from build123d import *

# Parameters (mm, degrees)
F0_R         = 1.8
F0_R_2       = 13.5
F0_W         = 20.1372796029
F0_H         = 13.5
F1_DEPTH     = 2
F2_W         = 3
F2_H         = 33.5
F3_DEPTH     = 27
F4_W         = 16.1372796029
F4_H         = 3
F5_DEPTH     = 25
F6_R         = 1.8
F6_W         = 4
F6_H         = 11
F7_DEPTH     = 25
F8_SIZE      = 25
F9_SIZE      = 14
F10_R        = 5
F11_T1_DEPTH = 2
F11_T3_DEPTH = 32


# Not quite as in the source:
# - a fillet or chamfer that OpenCascade refuses, or shapes differently, is made with other operations: its cross-section is extruded or revolved along the edge and cut away or added


with BuildPart() as f1:
    # F0 (on Top) → F1 (new body)
    with BuildSketch(Plane.XY):
        Polygon((21.15, -21.15), (21.15, 21.15), (-21.15, 21.15), (-21.15, -1.15), (-21.15, -21.15), align=None)
        with Locations((-15.5, -15.5)):
            Circle(F0_R, mode=Mode.SUBTRACT)
        with Locations((15.5, -15.5)):
            Circle(F0_R, mode=Mode.SUBTRACT)
        with Locations((-15.5, 15.5)):
            Circle(F0_R, mode=Mode.SUBTRACT)
        Circle(F0_R_2, mode=Mode.SUBTRACT)
        with Locations((15.5, 15.5)):
            Circle(F0_R, mode=Mode.SUBTRACT)
        Polygon((-21.15, -21.15), (-21.15, -1.15), (-41.3, -1.15), (-41.3, -21.15), (-21.1627203971, -21.15), align=None)
        with Locations((-31.2313601986, -27.9)):
            Rectangle(F0_W, F0_H)
    extrude(amount=F1_DEPTH)

    # F2 (on Top) → F3 (join)
    with BuildSketch(Plane.XY):
        with Locations((-23.6627203971, -17.9)):
            Rectangle(F2_W, F2_H)
    extrude(amount=F3_DEPTH)

    # F4 (on face) → F5 (join)
    with BuildSketch(Plane.XY.offset(2)):
        with Locations((-33.2313601986, -33.15)):
            Rectangle(F4_W, F4_H)
    extrude(amount=F5_DEPTH)

    # F6 (on face) → F7 (cut)
    with BuildSketch(Plane(origin=(0, -31.65, 0), x_dir=(-1, 0, 0), z_dir=(0, 1, 0))):
        with Locations((35.5, 14.5)):
            Circle(F6_R)
        with Locations((35.5, 5.5)):
            Circle(F6_R)
        with Locations((35.5, 23.5)):
            Circle(F6_R)
        with Locations((28.2, 14.5)):
            Rectangle(F6_W, F6_H)
    extrude(amount=-F7_DEPTH, mode=Mode.SUBTRACT)

    # F8
    f8_edges = [f1.edges().sort_by_distance(p)[0] for p in [
        (-23.66272, -1.15, 27),
    ]]
    chamfer(f8_edges, length=F8_SIZE)

    # F9
    f9_edges = [f1.edges().sort_by_distance(p)[0] for p in [
        (-41.3, -1.15, 1),
    ]]
    chamfer(f9_edges, length=F9_SIZE)

    # F10
    f10_edges = [f1.edges().sort_by_distance(p)[0] for p in [
        (-41.3, -15.15, 1),
        (-27.3, -1.15, 1),
        (-21.16272, -34.65, 1),
        (-41.3, -33.15, 27),
    ]]
    fillet(f10_edges, radius=F10_R)

    # F11: fillet of radius 6 on 5 edges, made by hand

    # F11_s2 → F11_t1 (join)
    with BuildSketch(Plane.XY):
        with BuildLine():
            ThreePointArc((-26.1021448299, -1.2268404777), (-22.5517867046, 0.826546392), (-21.15, 4.6809509491))
            Line((-21.15, 4.6809509491), (-20.55, 4.6809509491))
            Line((-20.55, 4.6809509491), (-20.55, -1.15))
            Line((-20.55, -1.15), (-21.15, -1.75))
            ThreePointArc((-21.15, -1.75), (-25.2289321881, -1.75), (-25.9973593129, -1.8176196204))
            Line((-25.9973593129, -1.8176196204), (-26.1021448299, -1.2268404777))
        make_face()
        with BuildLine():
            ThreePointArc((-15.1627203971, -21.15), (-19.4053610842, -22.9073593129), (-21.1627203971, -27.15))
            Line((-21.1627203971, -27.15), (-21.1627203971, -21.15))
            Line((-21.1627203971, -21.15), (-15.1627203971, -21.15))
        make_face()
    extrude(amount=F11_T1_DEPTH)

    # F11_s4 → F11_t3 (cut)
    with BuildSketch(Plane.XY.offset(-15)):
        with BuildLine():
            ThreePointArc((21.15, -15.15), (19.3926406871, -19.3926406871), (15.15, -21.15))
            Line((15.15, -21.15), (21.15, -21.15))
            Line((21.15, -21.15), (21.15, -15.15))
        make_face()
        with BuildLine():
            ThreePointArc((15.15, 21.15), (19.3926406871, 19.3926406871), (21.15, 15.15))
            Line((21.15, 15.15), (21.15, 21.15))
            Line((21.15, 21.15), (15.15, 21.15))
        make_face()
        with BuildLine():
            ThreePointArc((-21.15, 15.15), (-19.3926406871, 19.3926406871), (-15.15, 21.15))
            Line((-15.15, 21.15), (-21.15, 21.15))
            Line((-21.15, 21.15), (-21.15, 15.15))
        make_face()
    extrude(amount=F11_T3_DEPTH, mode=Mode.SUBTRACT)


solid = f1.part
Here's how the part is built. I have some questions about the finished solid (model axes, mm). A direction names the side the tool comes from. Coordinates: 2 decimals unless noted, no trailing zeros. Write each loop counter-clockwise with the first axis right and the second up, starting at its lowest first coordinate (ties: lowest second). Pieces come first, ordered by that corner, then holes.
Item 1: I want a section at C-C on x = -35.5. Write out the boundary of the cut face in (y, z).
Item 2: Will these pins go through, and if not, where does the flat tip stop? pin 1 (5 mm diameter, centred on x = -5.5, y = -24.5, fed in from +Z); pin 2 (0.6 mm diameter, centred on y = 8, z = 1, fed in from -X); pin 3 (2.5 mm diameter, centred on y = -33, z = 13, fed in from +X); pin 4 (6 mm diameter, centred on x = -35.5, z = 5.5, fed in from +Y).
Item 3: If we mould it in two halves opening along Y, with no side actions, what happens to faces 1 (the cylindrical face through (16.468, -13.982, 0.986)), 2 (the flat face through (-33, -31.65, 14)), 3 (the cylindrical face through (-39.87, -33.13, 25.5))? For each: +Y half, -Y half, draft (parallel to the pull), parting line (faces both ways), or undercut.
Item 4: I want a section at D-D on y = 6. Write out the boundary of the cut face in (x, z), and give its area (3 significant figures).
Item 5: I want a section at A-A on x = 0. Write out the boundary of the cut face in (y, z), and give its area (3 significant figures).
Item 6: On a 3-axis mill with a long thin cutter (end or side, diameter ignored), from which of +Z, -Z, +X, -X, +Y, -Y can I reach the whole of each face in a straight line? I mean faces 4 (the flat face through (-10, -11, 2)), 5 (the flat face through (-28, -33, 20)), 6 (the flat face through (-21.163, -28, 1)). Say none if no direction works.
Item 7: If I drill on line 1 (Z direction, x = -35.5, y = -32.3); line 2 (Y direction, x = 15.5, z = 0.65); line 3 (Y direction, x = -34, z = 10.5), over which ranges is the centre line in solid material (lowest first)?
Findings below:
1. outline: (-34.65, 0) - (-9.35, 0) - (-9.35, 2) - (-31.65, 2) - (-31.65, 3.7) - (-34.65, 3.7) - close; (-34.65, 7.3) - (-31.65, 7.3) - (-31.65, 12.7) - (-34.65, 12.7) - close; (-34.65, 16.3) - (-31.65, 16.3) - (-31.65, 21.7) - (-34.65, 21.7) - close; (-34.65, 25.3) - (-31.65, 25.3) - (-31.65, 27) - (-34.65, 27) - close
2. pin 1: passes through
2. pin 2: stops at x = -21.15
2. pin 3: stops at x = -22.16
2. pin 4: stops at y = -31.65
3. face 1: undercut
3. face 2: +Y half
3. face 3: draft
4. outline: (-21.15, 0) - (-12.09, 0) - (-12.09, 2) - (-21.15, 2) - close; (12.09, 0) - (21.15, 0) - (21.15, 2) - (12.09, 2) - close
4. area: 36.2 mm2
5. outline: (-21.15, 0) - (-13.5, 0) - (-13.5, 2) - (-21.15, 2) - close; (13.5, 0) - (21.15, 0) - (21.15, 2) - (13.5, 2) - close
5. area: 30.6 mm2
6. face 4: +Z, +Y
6. face 5: +Y, -Y
6. face 6: +Z, -Z, +X, -Y
7. line 1: z = 0 to 3.7, 7.3 to 12.7, 16.3 to 21.7, 25.3 to 27
7. line 2: y = -21.14 to -17.3, -13.7 to 13.7, 17.3 to 21.14
7. line 3: y = -34.65 to -31.65
